```python
from build123d import *

# Parameters (mm, degrees)
SKETCH1_W           = 431.8
SKETCH1_H           = 304.8
BOSS_EXTRUDE1_DEPTH = 133.35
CUT_EXTRUDE1_START  = 2.54
SKETCH2_W           = 426.72
SKETCH2_H           = 302.26
CUT_EXTRUDE1_DEPTH  = 128.27


with BuildPart() as part:
    # Sketch1 → Boss-Extrude1 (new body)
    with BuildSketch(Plane(origin=(0, 0, 0), x_dir=(1, 0, 0), z_dir=(0, 1, 0))):
        Rectangle(SKETCH1_W, SKETCH1_H)
    extrude(amount=BOSS_EXTRUDE1_DEPTH)

    # Sketch2 → Cut-Extrude1 (cut)
    with BuildSketch(Plane(origin=(0, 0, 0), x_dir=(1, 0, 0), z_dir=(0, 1, 0)).offset(CUT_EXTRUDE1_START)):
        with Locations((0, -1.27)):
            Rectangle(SKETCH2_W, SKETCH2_H)
    extrude(amount=CUT_EXTRUDE1_DEPTH, mode=Mode.SUBTRACT)


solid = part.part
```
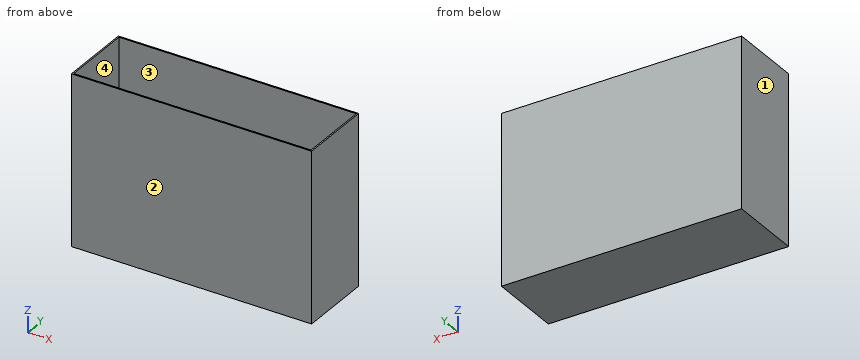
Geometry: final body of the model. Coordinates: model frame, mm. Face numbers are marked on the shaded views. Round coordinates to 2 decimals unless told otherwise and drop trailing zeros. Write each loop counter-clockwise with the first axis right and the second up, starting at its lowest first coordinate (ties: lowest second). Pieces come first, ordered by that corner, then holes.
Item 1: Pin query (flat end, axial travel): P1, Ø6, axis at x = 85.5, y = 114.5, coming from the +Z side. Return the tip coordinate at first contact, or that it passes through.
Item 2: Material intervals for L1, parallel to Y at x = 130, z = -90; L2, parallel to X at y = 18, z = 136; L3, parallel to Z at x = 37.5, y = 82, sorted ascending.
Item 3: Mould query, pull axis Y, two halves, no side actions, for the marked faces 1, 2, 3 and 4. Classes: +Y half, -Y half, draft (parallel to the pull), parting line (faces both ways), or undercut.
Item 4: Section query C-C (y = 67). Return loops of the section in (x, z), plus the area to 3 significant figures.
Item 5: Section query A-A (z = -40). Return loops of the section in (x, y), plus the area to 3 significant figures.
Item 6: Section query B-B (x = -158.5). Return loops of the section in (y, z), plus the area to 3 significant figures.
Completed:
1. P1: stops at z = -149.86
2. L1: y = 0 to 2.54, 130.81 to 133.35
2. L2: x = -215.9 to -213.36, 213.36 to 215.9
2. L3: z = -152.4 to -149.86
3. face 1: draft
3. face 2: -Y half
3. face 3: undercut
3. face 4: undercut
4. outline: (-215.9, -152.4) - (215.9, -152.4) - (215.9, 152.4) - (213.36, 152.4) - (213.36, -149.86) - (-213.36, -149.86) - (-213.36, 152.4) - (-215.9, 152.4) - close
4. area: 2,630 mm2
5. outline: (-215.9, 0) - (215.9, 0) - (215.9, 133.35) - (-215.9, 133.35) - close; hole (-213.36, 2.54) - (213.36, 2.54) - (213.36, 130.81) - (-213.36, 130.81) - close
5. area: 2,850 mm2
6. outline: (0, -152.4) - (133.35, -152.4) - (133.35, 152.4) - (130.81, 152.4) - (130.81, -149.86) - (2.54, -149.86) - (2.54, 152.4) - (0, 152.4) - close
6. area: 1,870 mm2
